```python
from build123d import *

# Parameters (mm, degrees)
BOSS_EXTRUDE1_DEPTH = 3
BOSS_EXTRUDE2_DEPTH = 2.6
BOSS_EXTRUDE3_DEPTH = 3
SKETCH8_R           = 1.8
CUT_EXTRUDE2_DEPTH  = 8


with BuildPart() as part:
    # Sketch1 → Boss-Extrude1 (new body)
    with BuildSketch(Plane.XY):
        with BuildLine():
            Line((-15.250000001, 13.250000001), (14.75, 13.250000001))
            ThreePointArc((14.75, 13.250000001), (15.457106781, 12.957106782), (15.75, 12.250000001))
            Line((15.75, 12.250000001), (15.75, -38.249999999))
            ThreePointArc((15.75, -38.249999999), (15.457106781, -38.95710678), (14.75, -39.249999999))
            Line((14.75, -39.249999999), (-15.250000001, -39.249999999))
            ThreePointArc((-15.250000001, -39.249999999), (-15.957106782, -38.95710678), (-16.250000001, -38.249999999))
            Line((-16.250000001, -38.249999999), (-16.250000001, 12.250000001))
            ThreePointArc((-16.250000001, 12.250000001), (-15.957106782, 12.957106782), (-15.250000001, 13.250000001))
        make_face()
    extrude(amount=BOSS_EXTRUDE1_DEPTH)

    # Sketch2 → Boss-Extrude2 (add)
    with BuildSketch(Plane.XY.offset(3)):
        with BuildLine():
            Line((15.75, -38.249999999), (15.75, -27.074999999))
            Line((15.75, -27.074999999), (-16.250000001, -27.074999999))
            Line((-16.250000001, -27.074999999), (-16.250000001, -38.249999999))
            ThreePointArc((-16.250000001, -38.249999999), (-15.957106782, -38.95710678), (-15.250000001, -39.249999999))
            Line((-15.250000001, -39.249999999), (14.75, -39.249999999))
            ThreePointArc((14.75, -39.249999999), (15.457106781, -38.95710678), (15.75, -38.249999999))
        make_face()
        with BuildLine():
            Line((14.75, 13.250000001), (-15.250000001, 13.250000001))
            ThreePointArc((-15.250000001, 13.250000001), (-15.957106782, 12.957106782), (-16.250000001, 12.250000001))
            Line((-16.250000001, 12.250000001), (-16.250000001, 3.075000001))
            Line((-16.250000001, 3.075000001), (15.75, 3.075000001))
            Line((15.75, 3.075000001), (15.75, 12.250000001))
            ThreePointArc((15.75, 12.250000001), (15.457106781, 12.957106782), (14.75, 13.250000001))
        make_face()
    extrude(amount=BOSS_EXTRUDE2_DEPTH)

    # Sketch7 → Boss-Extrude3 (add)
    with BuildSketch(Plane.XY.offset(3)):
        with BuildLine():
            Line((-14.732, 3.074800001), (14.732, 3.074800001))
            Line((14.732, 3.074800001), (15.875, 3.074800001))
            ThreePointArc((15.875, 3.074800001), (22.610192091, 0.284992092), (25.4, -6.450199999))
            Line((25.4, -6.450199999), (25.4, -17.549999999))
            ThreePointArc((25.4, -17.549999999), (22.610192091, -24.28519209), (15.875, -27.074999999))
            Line((15.875, -27.074999999), (14.732, -27.074999999))
            Line((14.732, -27.074999999), (-14.732, -27.074999999))
            Line((-14.732, -27.074999999), (-15.875, -27.074999999))
            ThreePointArc((-15.875, -27.074999999), (-22.610192091, -24.28519209), (-25.4, -17.549999999))
            Line((-25.4, -17.549999999), (-25.4, -6.450199999))
            ThreePointArc((-25.4, -6.450199999), (-22.610192091, 0.284992092), (-15.875, 3.074800001))
            Line((-15.875, 3.074800001), (-14.732, 3.074800001))
        make_face()
    extrude(amount=-BOSS_EXTRUDE3_DEPTH)

    # Sketch8 → Cut-Extrude2 (cut)
    with BuildSketch(Plane.XY):
        with Locations((0, 7)):
            Circle(SKETCH8_R)
        with Locations((0, -31)):
            Circle(SKETCH8_R)
    extrude(amount=CUT_EXTRUDE2_DEPTH, mode=Mode.SUBTRACT)


solid = part.part
```
Geometry check sheet. Reference: the model listing, model coordinates, mm. A direction names the side the tool comes from. Give positions to 0.01 mm unless a question says otherwise; leave off trailing zeros. Loops run counter-clockwise (first coordinate to the right, second up) from the corner with the lowest first, then second, coordinate; pieces in that order, holes last. Notation, with made-up numbers: M -28.5,84 L -1.5,84 A27 ccw -1.5,101 Z; hole C 53.5,5 d4. An arc over 180 degrees is marked long. Write item = value, one per line.
(1) Material ranges on line 1 (Y direction, x = 0, z = 1.8); line 2 (Y direction, x = 0, z = 4.05) (3 decimals); line 3 (Y direction, x = -10.5, z = 3.9) (3 decimals), recorded low to high. Write a range as [from, to].
Answer below:
line_1 = [-39.25, -32.8], [-29.2, 5.2], [8.8, 13.25]
line_2 = [-39.25, -32.8], [-29.2, -27.075], [3.075, 5.2], [8.8, 13.25]
line_3 = [-39.25, -27.075], [3.075, 13.25]
(2) Sectioned sample at D-D, the plane x = 13. Record the cut outline in (y, z) (3 decimals), plus the area to 3 significant figures.
Answer below:
outline = M -39.25,0 L 13.25,0 L 13.25,5.6 L 3.075,5.6 L 3.075,3 L -27.075,3 L -27.075,5.6 L -39.25,5.6 Z
area = 216 mm2
(3) Sectioned sample at C-C, the plane x = 0. Record the cut outline in (y, z) (3 decimals), plus the area to 3 significant figures.
Answer below:
outline = M -39.25,0 L -32.8,0 L -32.8,5.6 L -39.25,5.6 Z; M -29.2,0 L 5.2,0 L 5.2,5.6 L 3.075,5.6 L 3.075,3 L -27.075,3 L -27.075,5.6 L -29.2,5.6 Z; M 8.8,0 L 13.25,0 L 13.25,5.6 L 8.8,5.6 Z
area = 175 mm2
(4) Sectioned sample at B-B, the plane y = -31. Record the cut outline in (x, z), plus the area to 3 significant figures.
Answer below:
outline = M -16.25,0 L -1.8,0 L -1.8,5.6 L -16.25,5.6 Z; M 1.8,0 L 15.75,0 L 15.75,5.6 L 1.8,5.6 Z
area = 159 mm2
(5) Release check for a two-part mould opening along Y. For faces 6 (the face through (0, -39.25, 3)), 7 (the face through (-0.234, -29.215, 2.761)), 8 (the face through (0, 9, 5.6)) record: released by +Y, released by -Y, zero draft, split by the parting line, or undercut.
Answer below:
face_6 = released by -Y
face_7 = undercut
face_8 = zero draft
(6) Tool access check on faces 1 (the face through (22.684, -24.211, 1.521)), 2 (the face through (-16.25, 8, 3)), 3 (the face through (-16.25, -33, 3)), 4 (the face through (15.75, 8, 3)), 5 (the face through (0, -12, 3)). Record the directions out of +Z, -Z, +X, -X, +Y, -Y that give a thin tool (end or side, any length) a straight path to the whole face; none if there is none.
Answer below:
face_1 = +Z, -Z, +X, -Y
face_2 = +Z, -Z, -X, +Y
face_3 = +Z, -Z, -X, -Y
face_4 = +Z, -Z, +X, +Y
face_5 = +Z, +X, -X
(7) Sectioned sample at A-A, the plane z = 4.6. Record the cut outline in (x, y) (3 decimals).
Answer below:
outline = M -16.25,-38.25 A1 ccw -15.25,-39.25 L 14.75,-39.25 A1 ccw 15.75,-38.25 L 15.75,-27.075 L -16.25,-27.075 Z; M -16.25,3.075 L 15.75,3.075 L 15.75,12.25 A1 ccw 14.75,13.25 L -15.25,13.25 A1 ccw -16.25,12.25 Z; hole C 0,-31 d3.6; hole C 0,7 d3.6
(8) Gauge pin test, flat ends, axial feed: pin 1 Ø2 at (y, z) = (2, 0.5) entering from +X; pin 2 Ø1.7 at (y, z) = (-30.5, 2.5) entering from -X; pin 3 Ø9 at (x, y) = (-12, -15.5) entering from +Z. Record the tip position at first contact, or that the pin passes through.
Answer below:
pin_1 = 21.81
pin_2 = -16.25
pin_3 = 3
